```python
from build123d import *

# Parameters (mm, degrees)
SKETCH1_R           = 50
BOSS_EXTRUDE1_DEPTH = 6.2
SKETCH2_R           = 5.5
CUT_EXTRUDE1_DEPTH  = 71.981969542
SKETCH3_R           = 1.4
CUT_EXTRUDE2_DEPTH  = 71.981969542
SKETCH4_R           = 3.1
CUT_EXTRUDE3_DEPTH  = 71.981969542


with BuildPart() as part:
    # Sketch1 → Boss-Extrude1 (new body)
    with BuildSketch(Plane.XY):
        with Locations(Location((0, 0, 0), (0, 0, 180))):
            Circle(SKETCH1_R)
    extrude(amount=BOSS_EXTRUDE1_DEPTH)

    # Sketch2 → Cut-Extrude1 (cut, through all)
    with BuildSketch(Plane(origin=(0, 0, 0), x_dir=(-1, 0, 0), z_dir=(0, 0, -1))):
        Circle(SKETCH2_R)
    extrude(amount=-CUT_EXTRUDE1_DEPTH, mode=Mode.SUBTRACT)

    # Sketch3 → Cut-Extrude2 (cut, through all)
    with BuildSketch(Plane(origin=(0, 0, 0), x_dir=(-1, 0, 0), z_dir=(0, 0, -1))):
        with Locations((8.1, 0)):
            Circle(SKETCH3_R)
        with Locations((-4.05, -7.014805771)):
            Circle(SKETCH3_R)
        with Locations((-4.05, 7.014805771)):
            Circle(SKETCH3_R)
    extrude(amount=-CUT_EXTRUDE2_DEPTH, mode=Mode.SUBTRACT)

    # Sketch4 → Cut-Extrude3 (cut, through all)
    with BuildSketch(Plane(origin=(0, 0, 0), x_dir=(-1, 0, 0), z_dir=(0, 0, -1))):
        with Locations((42, 0)):
            Circle(SKETCH4_R)
        with Locations((29.69848481, -29.69848481)):
            Circle(SKETCH4_R)
        with Locations((0, -42)):
            Circle(SKETCH4_R)
        with Locations((-29.69848481, -29.69848481)):
            Circle(SKETCH4_R)
        with Locations((-42, 0)):
            Circle(SKETCH4_R)
        with Locations((-29.69848481, 29.69848481)):
            Circle(SKETCH4_R)
        with Locations((0, 42)):
            Circle(SKETCH4_R)
        with Locations((29.69848481, 29.69848481)):
            Circle(SKETCH4_R)
    extrude(amount=-CUT_EXTRUDE3_DEPTH, mode=Mode.SUBTRACT)


solid = part.part
```
Build history of the part. All positions in model axes, mm. Coordinates: 2 decimals unless noted, no trailing zeros. Order: outer loops, then holes, each group sorted by start corner. A loop starts at its lowest first (then second) coordinate and runs counter-clockwise, first axis right, second up. Notation, with made-up numbers: (11.25, -30) -> (22.25, -30) arc R22 ccw to (22.25, 0) -> close; hole circle Ø2 at (-6.75, 36.5). An arc over 180 degrees is marked (long way). Answer in a Markdown table with one row per item. Add a question column.
Q1. Band-saw the part on A-A, the plane x = 0. List the corners of the cut face in (y, z).
Q2. Band-saw the part on D-D, the plane y = -42. List the corners of the cut face in (x, z), then the cut area to 3 significant figures.
Q3. Band-saw the part on C-C, the plane z = 2.75. Give the number of separate pieces and of enclosed holes in the cut face, then the cut area to 3 significant figures.
Q4. Wall check: line 1 along Y through (x, z) = (0, 4); line 2 along X through (y, z) = (-2.5, 3); line 3 along Y through (x, z) = (-32.5, 2.25). Give the ranges that are in metal, low to high. Write a range as [from, to].
Q5. Drop flat-ended pins along their axis: pin 1 (10 mm diameter, centred on x = 0, y = -42, fed in from +Z); pin 2 (1.5 mm diameter, centred on x = -19, z = 4.5, fed in from +Y). Give the stop position or say it passes through.
Q6. Band-saw the part on B-B, the plane x = 43. List the corners of the cut face in (y, z).
Q7. Mould opens along Y. For faces 1 (the face through (-47.69, -15.02, 3.06)), 2 (the face through (3.297, 8.195, 3.057)), 3 (the face through (1, 10, 0)) say: +Y half, -Y half, draft (parallel to the pull), parting line (faces both ways), or undercut.
Answers follow:
| question | item | result |
|---|---|---|
| 1 | outline | (-50, 0) -> (-45.1, 0) -> (-45.1, 6.2) -> (-50, 6.2) -> close; (-38.9, 0) -> (-5.5, 0) -> (-5.5, 6.2) -> (-38.9, 6.2) -> close; (5.5, 0) -> (38.9, 0) -> (38.9, 6.2) -> (5.5, 6.2) -> close; (45.1, 0) -> (50, 0) -> (50, 6.2) -> (45.1, 6.2) -> close |
| 2 | outline | (-27.13, 0) -> (-3.1, 0) -> (-3.1, 6.2) -> (-27.13, 6.2) -> close; (3.1, 0) -> (27.13, 0) -> (27.13, 6.2) -> (3.1, 6.2) -> close |
| 2 | area | 298 mm^2 |
| 3 | separate pieces | 1 |
| 3 | enclosed holes | 12 |
| 3 | area | 7,500 mm^2 |
| 4 | line 1 | [-50, -45.1], [-38.9, -5.5], [5.5, 38.9], [45.1, 50] |
| 4 | line 2 | [-49.94, -43.83], [-40.17, -4.9], [4.9, 40.17], [43.83, 49.94] |
| 4 | line 3 | [-38, -31.03], [-28.37, 28.37], [31.03, 38] |
| 5 | pin 1 | z = 6.2 |
| 5 | pin 2 | y = 46.55 |
| 6 | outline | (-25.51, 0) -> (-2.93, 0) -> (-2.93, 6.2) -> (-25.51, 6.2) -> close; (2.93, 0) -> (25.51, 0) -> (25.51, 6.2) -> (2.93, 6.2) -> close |
| 7 | face 1 | parting line |
| 7 | face 2 | undercut |
| 7 | face 3 | draft |
